Verification items for the finished model (mm, model axes). A direction names the side the tool comes from. Give positions to 0.01 mm unless a question says otherwise; leave off trailing zeros. Loops run counter-clockwise (first coordinate to the right, second up) from the corner with the lowest first, then second, coordinate; pieces in that order, holes last. Notation, with made-up numbers: (-22.75, 42) -> (6.25, 42) arc R6 cw to (6.25, 50) -> close; hole circle Ø10 at (-7, 23.5). An arc over 180 degrees is marked (long way). Use one line per item in the form item = value. Start each with the question number.
from build123d import *

# Parameters (mm, degrees)
SKETCH1_R           = 7.8
BOSS_EXTRUDE1_DEPTH = 5.5
SKETCH2_R           = 6
BOSS_EXTRUDE2_DEPTH = 8.5
SKETCH4_R           = 6
BOSS_EXTRUDE3_DEPTH = 16.5
SKETCH7_R           = 6
BOSS_EXTRUDE4_DEPTH = 8.2
SKETCH3_R           = 4
CUT_EXTRUDE2_DEPTH  = 41.241396596
SKETCH8_R           = 6
BOSS_EXTRUDE5_DEPTH = 9.4


with BuildPart() as part:
    # Sketch1 → Boss-Extrude1 (new body)
    with BuildSketch(Plane(origin=(0, 0, 0), x_dir=(1, 0, 0), z_dir=(0, 1, 0))):
        with Locations(Location((0, 0, 0), (0, 0, 270))):
            Circle(SKETCH1_R)
    extrude(amount=BOSS_EXTRUDE1_DEPTH)

    # Sketch2 → Boss-Extrude2 (add)
    with BuildSketch(Plane(origin=(0, 5.5, 0), x_dir=(1, 0, 0), z_dir=(0, 1, 0))):
        with Locations(Location((1, 0, 0), (0, 0, 270))):
            Circle(SKETCH2_R)
    extrude(amount=BOSS_EXTRUDE2_DEPTH)

    # Sketch4 → Boss-Extrude3 (add)
    with BuildSketch(Plane(origin=(0, 14, 0), x_dir=(1, 0, 0), z_dir=(0, 1, 0))):
        with Locations(Location((-0.5, 0.866025404, 0), (0, 0, 51.701078932))):
            Circle(SKETCH4_R)
    extrude(amount=BOSS_EXTRUDE3_DEPTH)

    # Sketch7 → Boss-Extrude4 (add)
    with BuildSketch(Plane(origin=(0, 30.5, 0), x_dir=(1, 0, 0), z_dir=(0, 1, 0))):
        with Locations(Location((-0.5, -0.866025404, 0), (0, 0, 8.298921068))):
            Circle(SKETCH7_R)
    extrude(amount=BOSS_EXTRUDE4_DEPTH)

    # Sketch3 → Cut-Extrude2 (cut, through all)
    with BuildSketch(Plane.XZ):
        with Locations(Location((0, 0, 0), (0, 0, 270))):
            Circle(SKETCH3_R)
    extrude(amount=-CUT_EXTRUDE2_DEPTH, mode=Mode.SUBTRACT)

    # Sketch8 → Boss-Extrude5 (add)
    with BuildSketch(Plane(origin=(0, 38.7, 0), x_dir=(1, 0, 0), z_dir=(0, 1, 0))):
        with Locations(Location((0, 0, 0), (0, 0, 154.780191847))):
            Circle(SKETCH8_R)
    extrude(amount=BOSS_EXTRUDE5_DEPTH)


solid = part.part
Item 1: Sectioned sample at D-D, the plane z = -4.5. Enter the section's corners in (x, y).
Item 2: Material ranges on line 1 (Y direction, x = 1.25, z = 5); line 2 (Y direction, x = -7, z = -2.5); line 3 (Y direction, x = -3.75, z = 4.25), recorded low to high.
Item 3: Sectioned sample at A-A, the plane z = 1.75. Enter the section's corners in (x, y).
Item 4: Gauge pin test, flat ends, axial feed: pin 1 Ø3 at (x, y) = (5.5, 29) entering from -Z; pin 2 Ø1.5 at (y, z) = (36, 6) entering from +X; pin 3 Ø1 at (x, y) = (3, 18.5) entering from +Z. Record the tip position at first contact, or that the pin passes through.
Item 5: Sectioned sample at C-C, the plane y = 33.5. Enter the section's corners in (x, z), and give its area (3 significant figures).
Item 6: Sectioned sample at B-B, the plane x = -0.5. Enter the section's corners in (y, z).
Item 7: Tool access check on faces 4 (the flat face through (-5.2, 5.5, 1.1)), 5 (the flat face through (0, 38.7, 0)), 6 (the flat face through (-0.3, 30.5, 5.3)). Record the directions out of +Z, -Z, +X, -X, +Y, -Y that give a thin tool (end or side, any length) a straight path to the whole face; none if there is none.
Item 8: Draft check along Z on faces 1 (the cylindrical face through (-1.3, 9.69, 5.54)), 2 (the cylindrical face through (-3.905, 19.079, 0.867)), 3 (the flat face through (-5, 14, -2)). Enter one of: +Z half, -Z half, draft (parallel to the pull), parting line (faces both ways), or undercut.
Outcome:
q1.outline = (-6.37, 0) -> (6.37, 0) -> (6.37, 5.5) -> (4.97, 5.5) -> (4.97, 14) -> (4.27, 14) -> (4.27, 30.5) -> (2.18, 30.5) -> (2.18, 38.7) -> (3.97, 38.7) -> (3.97, 48.1) -> (-3.97, 48.1) -> (-3.97, 38.7) -> (-3.18, 38.7) -> (-3.18, 30.5) -> (-5.27, 30.5) -> (-5.27, 14) -> (-2.97, 14) -> (-2.97, 5.5) -> (-6.37, 5.5) -> close
q2.line_1 = 0 to 14, 30.5 to 48.1
q2.line_2 = 0 to 5.5
q2.line_3 = 0 to 5.5, 30.5 to 48.1
q3.outline = (-7.6, 0) -> (-3.6, 0) -> (-3.6, 38.7) -> (3.6, 38.7) -> (3.6, 0) -> (7.6, 0) -> (7.6, 5.5) -> (6.74, 5.5) -> (6.74, 14) -> (4.9, 14) -> (4.9, 30.5) -> (5.43, 30.5) -> (5.43, 38.7) -> (5.74, 38.7) -> (5.74, 48.1) -> (-5.74, 48.1) -> (-5.74, 38.7) -> (-6.43, 38.7) -> (-6.43, 30.5) -> (-5.9, 30.5) -> (-5.9, 14) -> (-4.74, 14) -> (-4.74, 5.5) -> (-7.6, 5.5) -> close
q4.pin_1 = -4.83
q4.pin_2 = 3.6
q4.pin_3 = 4.33
q5.outline = circle Ø12 at (-0.5, 0.87); hole circle Ø8 at (0, 0)
q5.area = 62.8 mm^2
q6.outline = (0, -7.78) -> (5.5, -7.78) -> (5.5, -5.81) -> (14, -5.81) -> (14, -6.87) -> (30.5, -6.87) -> (30.5, -5.13) -> (38.7, -5.13) -> (38.7, -5.98) -> (48.1, -5.98) -> (48.1, 5.98) -> (38.7, 5.98) -> (38.7, 6.87) -> (30.5, 6.87) -> (30.5, 5.13) -> (14, 5.13) -> (14, 5.81) -> (5.5, 5.81) -> (5.5, 7.78) -> (0, 7.78) -> (0, 3.97) -> (38.7, 3.97) -> (38.7, -3.97) -> (0, -3.97) -> close
q7.face_4 = none
q7.face_5 = -Y
q7.face_6 = +Z
q8.face_1 = parting line
q8.face_2 = undercut
q8.face_3 = draft
